Geometry: final body of the model. Coordinates: model frame, mm. A direction names the side the tool comes from. Round coordinates to 2 decimals unless told otherwise and drop trailing zeros. Loops run counter-clockwise (first coordinate to the right, second up) from the corner with the lowest first, then second, coordinate; pieces in that order, holes last. Notation, with made-up numbers: (11.25, 46.5) - (21.25, 46.5) arc R22 ccw to (21.25, 56.5) - close; hole circle Ø9 at (-27, -28). An arc over 180 degrees is marked (long way). Use CSV: the item, a comma, the result in double quotes.
from build123d import *

# Parameters (mm, degrees)
F0_W      = 300
F0_H      = 174.4493450305
F1_DEPTH  = 2.794
F2_W      = 5
F2_H      = 5
F2_W_2    = 7
F2_H_2    = 7
F3_DEPTH  = 100
F4_W      = 30
F4_H      = 30
F5_DEPTH  = 79.6
F6_W      = 26
F6_H      = 59.6
F7_DEPTH  = 1.1
F9_DEPTH  = 4.8
F11_DEPTH = 100
F12_W     = 68
F12_H     = 5
F13_DEPTH = 100
F14_W     = 68
F14_H     = 5
F15_DEPTH = 100
F17_DEPTH = 100
F18_W     = 129.6291201784
F18_H     = 31.5
F18_H_2   = 25
F19_DEPTH = 16.5
F20_W     = 68
F20_H     = 31.5
F20_H_2   = 25
F21_DEPTH = 25
F22_W     = 68
F22_H     = 31.5
F22_H_2   = 25
F23_DEPTH = 25
F24_W     = 129.6291201784
F24_H     = 31.5
F24_H_2   = 25
F25_DEPTH = 25
F26_DEPTH = 100
F27_W     = 50
F27_H     = 16.5
F27_H_2   = 25
F27_H_3   = 6
F28_DEPTH = 1.3


with BuildPart() as f1:
    # F0 (on Top) → F1 (new body)
    with BuildSketch(Plane.XY):
        Rectangle(F0_W, F0_H)
    extrude(amount=F1_DEPTH)

    # F2 (on face) → F3 (join)
    with BuildSketch(Plane.XY.offset(2.794)):
        with Locations((-142.5, -72.5)):
            Rectangle(F2_W, F2_H)
        with Locations((-92.5, 52.5)):
            Rectangle(F2_W, F2_H)
        with Locations((92.5, 52.5)):
            Rectangle(F2_W, F2_H)
        with Locations((142.5, -72.5)):
            Rectangle(F2_W, F2_H)
        with Locations((-18.5, 53.5)):
            Rectangle(F2_W_2, F2_H_2)
        with Locations((18.5, 53.5)):
            Rectangle(F2_W_2, F2_H_2)
        Polygon((-90, 60), (-90, 56.5), (-15, 58.5), (-15, 62), align=None)
        Polygon((90, 60), (15, 62), (15, 58.5), (90, 56.5), align=None)
        Polygon((96.0606601718, 56.0606601718), (146.02977278, -68.9093268035), (148.4921801752, -66.4220492114), (99.5606601718, 59.5606601718), align=None)
        Polygon((-96.0627255066, 56.0585908075), (-99.5627255066, 59.5562038535), (-148.5355339059, -66.4644660941), (-146.0606601718, -68.9393398282), align=None)
    extrude(amount=F3_DEPTH)

    # F4 (on face) → F5 (join)
    with BuildSketch(Plane.XY.offset(2.794)):
        with Locations((0, 56.6965335608)):
            Rectangle(F4_W, F4_H)
    extrude(amount=F5_DEPTH)

    # F6 (on face) → F7 (join)
    with BuildSketch(Plane.XZ.offset(-41.6965335608)):
        with Locations((0, 50.594)):
            Rectangle(F6_W, F6_H)
    extrude(amount=F7_DEPTH)

    # F8 (on face) → F9 (cut)
    with BuildSketch(Plane.XZ.offset(-41.6965335608)):
        with BuildLine():
            add(Edge.make_bspline(
                [(12.06954394, 11.794), (12.06954394, 19.7033991149), (-6.03477197, 15.7486995575), (-24.13908788, 11.794), (-6.03477197, 7.8393004425), (12.06954394, 3.8846008851), (12.06954394, 11.794)],
                knots=[0, 0, 0, 2.0943951024, 2.0943951024, 4.1887902048, 4.1887902048, 6.2831853072, 6.2831853072, 6.2831853072], degree=2, weights=[1, 0.5, 1, 0.5, 1, 0.5, 1]))
        make_face()
    extrude(amount=-F9_DEPTH, mode=Mode.SUBTRACT)

    # F10 (on face) → F11 (join)
    with BuildSketch(Plane.XY.offset(2.794)):
        Polygon((-140, -70), (-140, -75), (-90, 50), (-95, 50), (-95, 55), (-145, -70), align=None)
    extrude(amount=F11_DEPTH)

    # F12 (on face) → F13 (join)
    with BuildSketch(Plane.XY.offset(2.794)):
        with Locations((-56, 52.5)):
            Rectangle(F12_W, F12_H)
    extrude(amount=F13_DEPTH)

    # F14 (on face) → F15 (join)
    with BuildSketch(Plane.XY.offset(2.794)):
        with Locations((56, 52.5)):
            Rectangle(F14_W, F14_H)
    extrude(amount=F15_DEPTH)

    # F16 (on face) → F17 (join)
    with BuildSketch(Plane.XY.offset(2.794)):
        Polygon((90, 50), (140, -75), (140, -70), (145, -70), (95, 55), (95, 50), align=None)
    extrude(amount=F17_DEPTH)

    # F18 (on face) → F19 (cut)
    with BuildSketch(Plane(origin=(-94.8275862069, 37.9310344828, 0), x_dir=(0.3713906764, 0.9284766909, 0), z_dir=(0.9284766909, -0.3713906764, 0))):
        with Locations((-51.8158864168, 87.044)):
            Rectangle(F18_W, F18_H)
        with Locations((-51.8158864168, 52.794)):
            Rectangle(F18_W, F18_H_2)
        with Locations((-51.8158864168, 18.544)):
            Rectangle(F18_W, F18_H)
    extrude(amount=-F19_DEPTH, mode=Mode.SUBTRACT)

    # F20 (on face) → F21 (cut)
    with BuildSketch(Plane.XZ.offset(-50)):
        with Locations((-56, 87.044)):
            Rectangle(F20_W, F20_H)
        with Locations((-56, 52.794)):
            Rectangle(F20_W, F20_H_2)
        with Locations((-56, 18.544)):
            Rectangle(F20_W, F20_H)
    extrude(amount=-F21_DEPTH, mode=Mode.SUBTRACT)

    # F22 (on face) → F23 (cut)
    with BuildSketch(Plane.XZ.offset(-50)):
        with Locations((56, 18.544)):
            Rectangle(F22_W, F22_H)
        with Locations((56, 52.794)):
            Rectangle(F22_W, F22_H_2)
        with Locations((56, 87.044)):
            Rectangle(F22_W, F22_H)
    extrude(amount=-F23_DEPTH, mode=Mode.SUBTRACT)

    # F24 (on face) → F25 (cut)
    with BuildSketch(Plane(origin=(94.8275862069, 37.9310344828, 0), x_dir=(0.3713906764, -0.9284766909, 0), z_dir=(-0.9284766909, -0.3713906764, 0))):
        with Locations((51.8158864168, 87.044)):
            Rectangle(F24_W, F24_H)
        with Locations((51.8158864168, 52.794)):
            Rectangle(F24_W, F24_H_2)
        with Locations((51.8158864168, 18.544)):
            Rectangle(F24_W, F24_H)
    extrude(amount=-F25_DEPTH, mode=Mode.SUBTRACT)

    # F2 (on face) → F26 (join)
    with BuildSketch(Plane.XY.offset(2.794)):
        Polygon((-96.0627255066, 56.0585908075), (-99.5627255066, 59.5562038535), (-148.5355339059, -66.4644660941), (-146.0606601718, -68.9393398282), align=None)
        Polygon((-90, 60), (-90, 56.5), (-15, 58.5), (-15, 62), align=None)
        Polygon((90, 60), (15, 62), (15, 58.5), (90, 56.5), align=None)
        Polygon((96.0606601718, 56.0606601718), (146.02977278, -68.9093268035), (148.4921801752, -66.4220492114), (99.5606601718, 59.5606601718), align=None)
    extrude(amount=F26_DEPTH)

    # F27 (on face) → F28 (join)
    with BuildSketch(Plane(origin=(-94.8275862069, 37.9310344828, 0), x_dir=(0.3713906764, 0.9284766909, 0), z_dir=(0.9284766909, -0.3713906764, 0))):
        with Locations((-79.630446506, 79.544)):
            Rectangle(F27_W, F27_H)
        with Locations((-79.630446506, 52.794)):
            Rectangle(F27_W, F27_H_2)
        with Locations((-79.630446506, 68.294)):
            Rectangle(F27_W, F27_H_3)
        with Locations((-79.630446506, 26.044)):
            Rectangle(F27_W, F27_H)
        with Locations((-79.630446506, 37.294)):
            Rectangle(F27_W, F27_H_3)
        with Locations((-24.0013263276, 26.044)):
            Rectangle(F27_W, F27_H)
        with Locations((-24.0013263276, 37.294)):
            Rectangle(F27_W, F27_H_3)
        with Locations((-24.0013263276, 52.794)):
            Rectangle(F27_W, F27_H_2)
        with Locations((-24.0013263276, 68.294)):
            Rectangle(F27_W, F27_H_3)
        with Locations((-24.0013263276, 79.544)):
            Rectangle(F27_W, F27_H)
    extrude(amount=F28_DEPTH)


solid = f1.part
Item 1: Pin query (flat end, axial travel): P1, Ø1.2, axis at y = 41.5, z = 52, coming from the +X side; P2, Ø10, axis at y = -52.5, z = 75, coming from the +X side; P3, Ø4, axis at y = 41.5, z = 76, coming from the -X side. Return the tip coordinate at first contact, or that it passes through.
Final values:
P1,"stops at x = 106.81"
P2,"stops at x = 145.03"
P3,"stops at x = -107.36"
Item 2: Mould query, pull axis Z, two halves, no side actions, for faces 6 (the flat face through (38, 50, 67)), 7 (the flat face through (-93, 51.2, 52.6)), 8 (the flat face through (-142, -72, 102.794)), 9 (the flat face through (-117, -10, 40.294)). Classes: released by +Z, released by -Z, zero draft, split by the parting line, or undercut.
Final values:
face 6,"zero draft"
face 7,"undercut"
face 8,"released by +Z"
face 9,"undercut"
Item 3: Section A-A on y = 24. Give the number of separate pieces and of enclosed holes in the cut face, plus the area to 3 significant figures.
Final values:
separate pieces,"4"
enclosed holes,"0"
area,"2,000 mm²"
Item 4: Material intervals for line 1 (X direction, y = 52, z = 82.5); line 2 (X direction, y = 20, z = 26); line 3 (X direction, y = -51.5, z = 72), sorted ascending.
Final values:
line 1,"x = -102.5 to -97.69, -95 to -90, -22 to -15, 15 to 22, 90 to 95, 97.68 to 102.5"
line 2,"x = -114.93 to -110.49, -102 to -100.6, 110.48 to 114.93"
line 3,"x = -142.72 to -139.09, -130.6 to -129.2, 139.07 to 142.7"
Item 5: Section B-B on x = 55. Return the cut outline in (y, z).
Final values:
outline,"(-87.22, 0) - (87.22, 0) - (87.22, 2.79) - (60.93, 2.79) - (60.93, 102.79) - (57.43, 102.79) - (57.43, 2.79) - (-87.22, 2.79) - close; (50, 34.29) - (55, 34.29) - (55, 40.29) - (50, 40.29) - close; (50, 65.29) - (55, 65.29) - (55, 71.29) - (50, 71.29) - close"
Item 6: Reachability of faces 1 (the flat face through (18, 54, 102.794)), 2 (the flat face through (18, 57, 52)), 3 (the flat face through (-103, 15, 17.794)), 4 (the flat face through (0, 40.597, 51)), 5 (the flat face through (-104, 15, 26)) from +Z, -Z, +X, -X, +Y, -Y: full face, straight path, thin tool, end or side. Return the list, or none.
Final values:
face 1,"+Z, +X, -X, +Y, -Y"
face 2,"+Z"
face 3,"-Y"
face 4,"+Z, -Y"
face 5,"none"
